Here's the drawing with two shaded views (mm, measured from the low corner). I have some questions. A direction names the side the tool comes from. Round coordinates to 2 decimals unless told otherwise and drop trailing zeros. Loops run counter-clockwise (first coordinate to the right, second up) from the corner with the lowest first, then second, coordinate; pieces in that order, holes last. Notation, with made-up numbers: (-19, -27) - (-11, -27) arc R23 cw to (-11, 2) - close; hole circle Ø2 at (-26, 8.5). An arc over 180 degrees is marked (long way). Answer as CSV lines item,"result".
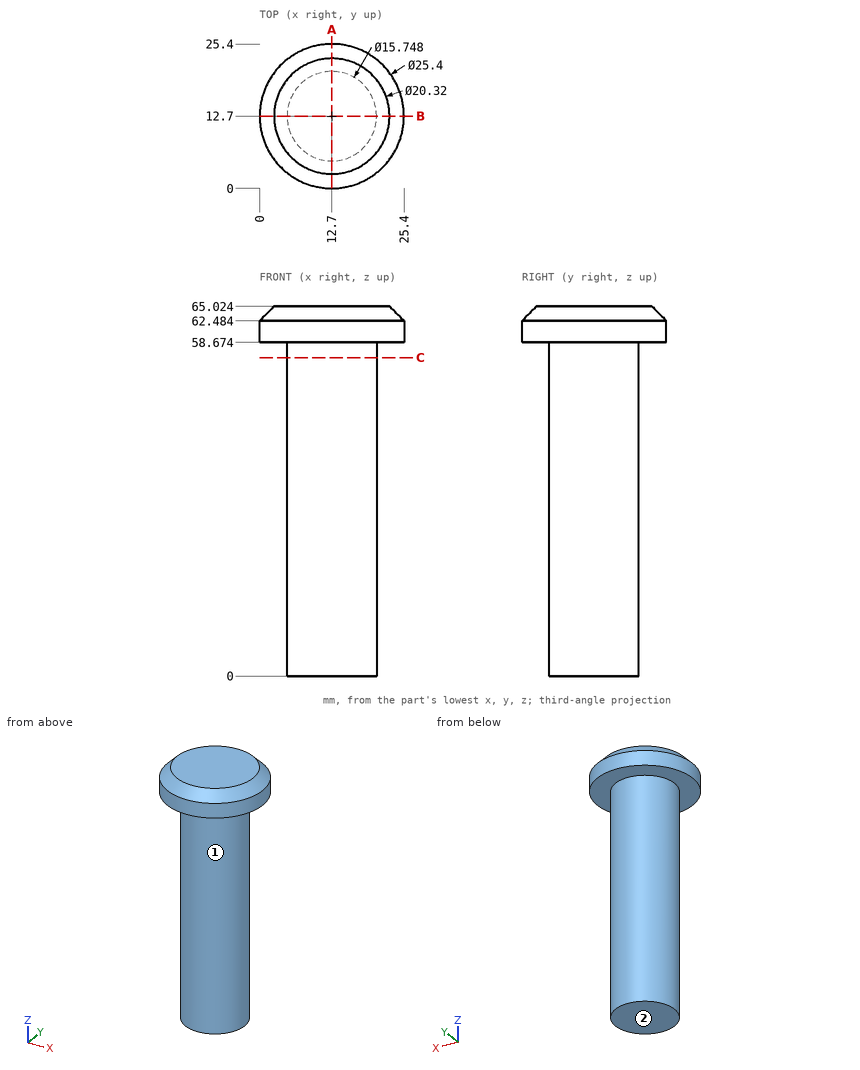
Q1. Imagine slicing it at C-C (z = 56). Write out the boundary of the cut face in (x, y).
Checks:
outline,"circle Ø15.75 at (12.7, 12.7)"
Q2. On a 3-axis mill with a long thin cutter (end or side, diameter ignored), from which of +Z, -Z, +X, -X, +Y, -Y can I reach the whole of each face in a straight line? I mean the marked faces 1 and 2. Say none if no direction works.
Checks:
face 1,"-Z"
face 2,"-Z, +X, -X, +Y, -Y"
Q3. I'm going to push flat-ended pins straight in: pin 1 Ø4 at (x, y) = (2.5, 4) entering from +Z; pin 2 Ø6 at (y, z) = (6.5, 24.5) entering from -X; pin 3 Ø2 at (y, z) = (12, 35.5) entering from +X. Where does each tip first touch, or does it pass through?
Checks:
pin 1,"z = 63.78"
pin 2,"x = 5.51"
pin 3,"x = 20.57"
Q4. If I drill on line 1 along Z through (x, y) = (6.25, 7.5); line 2 along Y through (x, z) = (13, 40); line 3 along X through (y, z) = (17.25, 37.5), over which ranges is the centre line in solid material (lowest first)? Write a range as [from, to].
Checks:
line 1,"[58.67, 65.02]"
line 2,"[4.83, 20.57]"
line 3,"[6.27, 19.13]"
Q5. Imagine slicing it at A-A (x = 12.7). Write out the boundary of the cut face in (y, z), then the cut area to 3 significant figures.
Checks:
outline,"(0, 58.67) - (4.83, 58.67) - (4.83, 0) - (20.57, 0) - (20.57, 58.67) - (25.4, 58.67) - (25.4, 62.48) - (22.86, 65.02) - (2.54, 65.02) - (0, 62.48) - close"
area,"1,080 mm²"
